CAD build for the part. Positions are in the model's coordinates, mm. Give positions to 0.01 mm unless a question says otherwise; leave off trailing zeros. Loops run counter-clockwise (first coordinate to the right, second up) from the corner with the lowest first, then second, coordinate; pieces in that order, holes last.
```python
from build123d import *

# Parameters (mm, degrees)
SKETCH_1_W             = 112
SKETCH_1_H             = 110.77381068
SKETCH_1_R             = 5.25
SM_BASE_FLANGE_1_DEPTH = 5
CHAMFER_1_SIZE         = 15


# Sheet-metal steps are written as plain solids
with BuildPart() as part:
    # Sketch 1 → Базовая кромка1 (new body)
    with BuildSketch(Plane.XY):
        with Locations((0, 58.38690534)):
            Rectangle(SKETCH_1_W, SKETCH_1_H)
        with Locations((-28, 73.77381068)):
            Circle(SKETCH_1_R, mode=Mode.SUBTRACT)
        with Locations((-28, 43)):
            Circle(SKETCH_1_R, mode=Mode.SUBTRACT)
        with Locations(Location((28, 73.77381068, 0), (0, 0, 180))):
            Circle(SKETCH_1_R, mode=Mode.SUBTRACT)
        with Locations(Location((28, 43, 0), (0, 0, 180))):
            Circle(SKETCH_1_R, mode=Mode.SUBTRACT)
    extrude(amount=-SM_BASE_FLANGE_1_DEPTH)

    # Фаска1
    chamfer_1_edges = [part.edges().sort_by_distance(p)[0] for p in [
        (56, 3, -2.5),
        (-56, 3, -2.5),
        (-56, 113.77381068, -2.5),
        (56, 113.77381068, -2.5),
    ]]
    chamfer(chamfer_1_edges, length=CHAMFER_1_SIZE)


solid = part.part
```
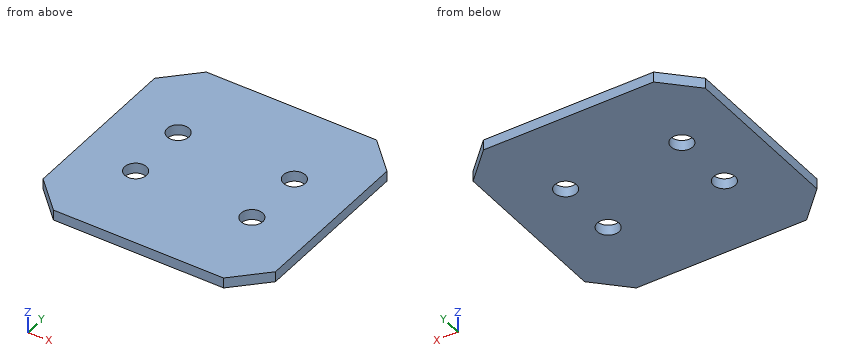
1. Saw through at A-A, the plane y = 43. List the corners of the cut face in (x, z), and give its area (3 significant figures).
Responses:
outline: (-56, -5) - (-33.25, -5) - (-33.25, 0) - (-56, 0) - close; (-22.75, -5) - (22.75, -5) - (22.75, 0) - (-22.75, 0) - close; (33.25, -5) - (56, -5) - (56, 0) - (33.25, 0) - close
area: 455 mm2
2. Saw through at B-B, the plane x = 28. List the corners of the cut face in (y, z), and give its area (3 significant figures).
Responses:
outline: (3, -5) - (37.75, -5) - (37.75, 0) - (3, 0) - close; (48.25, -5) - (68.52, -5) - (68.52, 0) - (48.25, 0) - close; (79.02, -5) - (113.77, -5) - (113.77, 0) - (79.02, 0) - close
area: 449 mm2
3. Saw through at C-C, the plane z = -3.5. List the corners of the cut face in (x, y).
Responses:
outline: (-56, 18) - (-41, 3) - (41, 3) - (56, 18) - (56, 98.77) - (41, 113.77) - (-41, 113.77) - (-56, 98.77) - close; hole circle Ø10.5 at (-28, 43); hole circle Ø10.5 at (-28, 73.77); hole circle Ø10.5 at (28, 43); hole circle Ø10.5 at (28, 73.77)
4. Probe line 1 along Y through (x, z) = (-28, -1.35); line 2 along X through (y, z) = (43.5, -4.7); line 3 along X through (y, z) = (78.5, -1.4). List the from-to ranges inside material, lowest first.
Responses:
line 1: y = 3 to 37.75, 48.25 to 68.52, 79.02 to 113.77
line 2: x = -56 to -33.23, -22.77 to 22.77, 33.23 to 56
line 3: x = -56 to -30.29, -25.71 to 25.71, 30.29 to 56
